Geometry check sheet. Reference: drawing and pictorial views, mm from the part's lowest x, y, z. A direction names the side the tool comes from. Round coordinates to 2 decimals unless told otherwise and drop trailing zeros. Write each loop counter-clockwise with the first axis right and the second up, starting at its lowest first coordinate (ties: lowest second). Pieces come first, ordered by that corner, then holes. Notation, with made-up numbers: M 51,60.5 L 94,60.5 A7 ccw 94,65.5 Z; hole C 74,13 d7. An arc over 180 degrees is marked long. Put each result on its own line as item: value. Start each with the question number.
(1) Section check D-D on x = 21. Record the cut outline in (y, z).
(2) Gauge pin test, flat ends, axial feed: pin 1 (12 mm diameter, centred on x = 200, y = 18, fed in from -Z); pin 2 (9 mm diameter, centred on y = 12, z = 21.5, fed in from -X); pin 3 (5 mm diameter, centred on x = 285, y = 8, fed in from -Z). Record the tip position at first contact, or that the pin passes through.
(3) Section check B-B on x = 285. Record the cut outline in (y, z), then the cut area to 3 significant figures.
(4) Section check C-C on y = 8. Record the cut outline in (x, z), then the cut area to 3 significant figures.
(5) Section check A-A on z = 8.5. Record the cut outline in (x, y), then the cut area to 3 significant figures.
(6) Material ranges on probe 1 along Y at (x, z) = (285, 7.25); probe 2 along X at (y, z) = (8, 7.25); probe 3 along X at (y, z) = (16, 15.5), recorded low to high.
(7) Tool access check on the marked faces 1 and 2. Record the directions out of +Z, -Z, +X, -X, +Y, -Y that give a thin tool (end or side, any length) a straight path to the whole face; none if there is none.
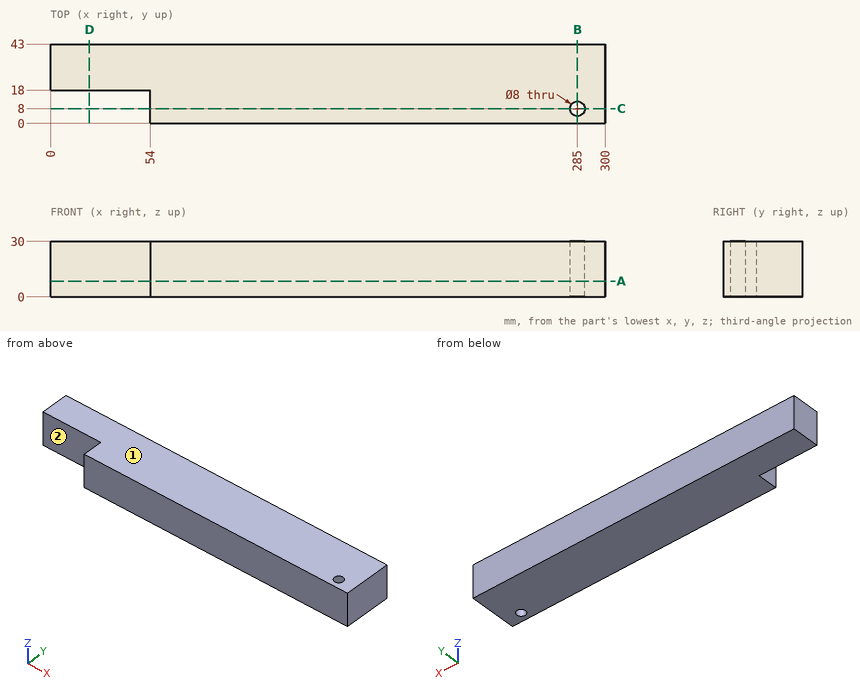
Answers follow:
1. outline: M 18,0 L 43,0 L 43,30 L 18,30 Z
2. pin 1: stops at z = 0
2. pin 2: stops at x = 54
2. pin 3: passes through
3. outline: M 0,0 L 4,0 L 4,30 L 0,30 Z; M 12,0 L 43,0 L 43,30 L 12,30 Z
3. area: 1,050 mm^2
4. outline: M 54,0 L 281,0 L 281,30 L 54,30 Z; M 289,0 L 300,0 L 300,30 L 289,30 Z
4. area: 7,140 mm^2
5. outline: M 0,18 L 54,18 L 54,0 L 300,0 L 300,43 L 0,43 Z; hole C 285,8 d8
5. area: 11,900 mm^2
6. probe 1: y = 0 to 4, 12 to 43
6. probe 2: x = 54 to 281, 289 to 300
6. probe 3: x = 54 to 300
7. face 1: +Z, +X, -X, +Y, -Y
7. face 2: +Z, -Z, -X, -Y
